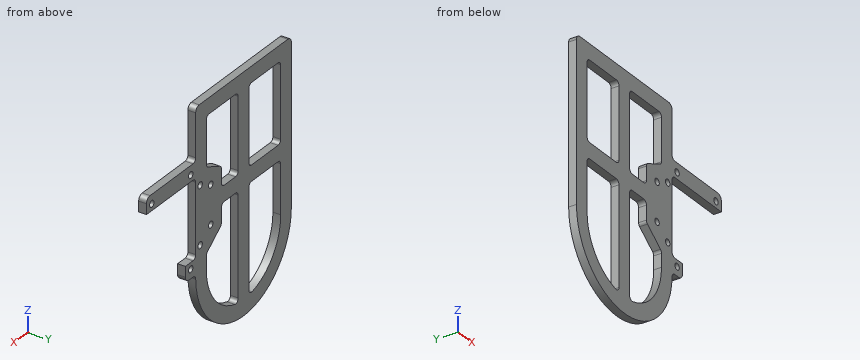
Autodesk Inventor part; units mm, degrees
ref_plane "YZ Plane" through (0, 0, 0) normal (1, 0, 0) x (0, 1, 0)
ref_plane "XZ Plane" through (0, 0, 0) normal (0, 1, 0) x (-1, 0, 0)
ref_plane "XY Plane" through (0, 0, 0) normal (0, 0, 1) x (1, 0, 0)
sketch "Sketch1" plane through (0, 0, 0) normal (0, 1, 0) x (-1, 0, 0)
  line L0 (0, 0) -> (0, -14.8)
  line L1 (0, -14.8) -> (-5.8, -14.8)
  line L2 (-5.8, -14.8) -> (-5.8, -20.8)
  line L3 (-5.8, -20.8) -> (0, -20.8)
  line L4 (0, 0) -> (0, 14.8)
  line L5 (0, 14.8) -> (-27.8, 14.8)
  line L6 (-27.8, 14.8) -> (-27.8, 20.8)
  line L7 (-27.8, 20.8) -> (0, 20.8)
  line L8 (0, 20.8) -> (0, 40.8)
  line L9 (0, 40.8) -> (54, 40.8)
  line L10 (0, -20.8) -> (0, -21.8)
  line L11 (54, 40.8) -> (54, -21.8)
  arc A0 (0, -21.8) -> (54, -21.8) centre (27, -21.8) ccw
  line L12 (-27.8, 17.3) -> (2.5, 17.3) construction
  line L13 (2.5, 17.3) -> (2.5, -17.3) construction
  line L14 (2.5, -17.3) -> (-5.8, -17.3) construction
  line L15 (0, 0) -> (2.5, 0) construction
  line L16 (2.5, 0) -> (8.5, 0) construction
  line L17 (8.5, -6.35) -> (8.5, 8.35) construction
  line L18 (-27.8, 14.8) -> (-5.8, -14.8) construction
  line L19 (-16.8, 0) -> (-21.8, 0) construction
  point P0 (-2.8, -17.3)
  point P1 (-2.8, 17.3)
  point P2 (-24.8, 17.3)
  point P3 (2.5, 11)
  point P4 (2.5, -11)
  dimension "d0" = 20
  dimension "d1" = 6
  dimension "d2" = 6
  dimension "d4" = 54
  dimension "d5" = 1
  dimension "d7" = 2.5
  dimension "d8" = 2.5
  dimension "d9" = 5.3
  dimension "d10" = 3
  dimension "d11" = 34.6
  dimension "d12" = 11
  dimension "d13" = 11
  dimension "d14" = 5.3
  dimension "d15" = 22
  dimension "d16" = 3
  dimension "d19" = 6
  dimension "d20" = 14.7
  dimension "d21" = 6.35
  dimension "d53" = 5
extrude "Extrusion1" add sketch "Sketch1" along normal blind 3
hole "Hole1" at (2.8, 0, -17.3) at (2.8, 0, 17.3) at (24.8, 0, 17.3) at (-2.5, 0, 11) at (-2.5, 0, -11) at (-8.5, 0, 8.35) at (-8.5, 0, -6.35) direction (0, 1, 0) diameter 2.5 end through all
fillet "ManufacturingFillet" radius 1.5 4 edges at (0, 1.5, -20.8) (0, 1.5, -14.8) (0, 1.5, 14.8) (0, 1.5, 20.8)
fillet "Fillet2" radius 2 4 edges at (5.8, 1.5, -20.8) (27.8, 1.5, 20.8) (0, 1.5, 40.8) (-54, 1.5, 40.8)
sketch "InteriorSketch" plane through (0, 3, 0) normal (0, 1, 0) x (1, 0, 0)
  arc A0 (-54, -38.8) -> (-52, -40.8) centre (-52, -38.8) ccw
  line L0 (-52, -40.8) -> (-2, -40.8)
  arc A1 (-2, -40.8) -> (0, -38.8) centre (-2, -38.8) ccw
  line L1 (0, -38.8) -> (0, -22.3)
  arc A2 (1.5, -20.8) -> (0, -22.3) centre (1.5, -22.3) ccw
  line L2 (1.5, -20.8) -> (25.8, -20.8)
  arc A3 (25.8, -20.8) -> (27.8, -18.8) centre (25.8, -18.8) ccw
  line L3 (27.8, -18.8) -> (27.8, -14.8)
  line L4 (27.8, -14.8) -> (1.5, -14.8)
  arc A4 (0, -13.3) -> (1.5, -14.8) centre (1.5, -13.3) ccw
  line L5 (0, -13.3) -> (0, 13.3)
  arc A5 (1.5, 14.8) -> (0, 13.3) centre (1.5, 13.3) ccw
  line L6 (1.5, 14.8) -> (5.8, 14.8)
  line L7 (5.8, 14.8) -> (5.8, 18.8)
  arc A6 (5.8, 18.8) -> (3.8, 20.8) centre (3.8, 18.8) ccw
  line L8 (3.8, 20.8) -> (1.4956, 20.8)
  arc A7 (-0.0042, 22.2737) -> (1.4956, 20.8) centre (1.4956, 22.3) ccw
  arc A8 (-0.0042, 22.2737) -> (-54, 21.8) centre (-27, 21.8) ccw
  line L9 (-54, 21.8) -> (-54, -38.8)
  circle A9 centre (-8.5, -8.35) radius 1.25
  circle A10 centre (-2.5, -11) radius 1.25
  circle A11 centre (2.8, -17.3) radius 1.25
  circle A12 centre (2.8, 17.3) radius 1.25
  circle A13 centre (24.8, -17.3) radius 1.25
  circle A14 centre (-2.5, 11) radius 1.25
  circle A15 centre (-8.5, 6.35) radius 1.25
  line L10 (-14.5, 9.2909) -> (-14.5, -12.2592)
  line L11 (-14.5, -12.2592) -> (-6, -16.0133)
  line L12 (-6, -16.0133) -> (-6, -34.8)
  line L13 (-6, -34.8) -> (-48, -34.8)
  circle A16 centre (-2.5, 11) radius 1.25 construction
  line L14 (-8.5, 6.35) -> (-2.5, 11) construction
  line L15 (-8.5, -8.35) -> (-2.5, -11) construction
  line L16 (-14.5, 9.2909) -> (-6, 15.8784)
  line L17 (-6, 15.8784) -> (-6, 21.8)
  line L18 (-6, 15.8784) -> (-6, 21.8)
  arc A17 (-6, 21.8) -> (-48, 21.8) centre (-27, 21.8) ccw
  line L19 (-48, 21.8) -> (-48, -34.8)
  line L20 (-6, 21.8) -> (-48, 21.8) construction
  line L21 (-27, -34.8) -> (-27, 42.8) construction
  line L22 (-14.5, -1.4841) -> (-48, -1.4841) construction
  line L23 (-14.5, 1.5159) -> (-24, 1.5159)
  line L24 (-24, 1.5159) -> (-24, 42.5846)
  line L25 (-30, 42.5846) -> (-30, 1.5159)
  line L26 (-30, 1.5159) -> (-48, 1.5159)
  line L27 (-48, -4.4841) -> (-30, -4.4841)
  line L28 (-30, -4.4841) -> (-30, -34.8)
  line L29 (-14.5, -4.4841) -> (-24, -4.4841)
  line L30 (-24, -4.4841) -> (-24, -34.8)
  line L31 (-30, 1.5159) -> (-24, 1.5159) construction
  line L32 (-30, 1.5159) -> (-30, -4.4841) construction
  point P0 (0, 0)
  point P1 (-14.5, -1.4841)
  point P2 (-27, -1.4841)
  point P3 (-30, -1.4841)
  point P4 (-27, 1.5159)
  dimension "d31" = 6
  dimension "d32" = 6
  dimension "d34" = 6
  dimension "d38" = 6
  dimension "d39" = 6
  dimension "d44" = 6
  dimension "d48" = 6
  dimension "d49" = 6
extrude "Extrusion3" cut sketch "InteriorSketch" against normal through all contours L10 L23 L24 A17 L17 L16 | L10 L11 L12 L13 L30 L29 | L25 L26 L19 A17 | L13 L19 L27 L28
fillet "Fillet3" radius 1.5 18 edges at (-24, 1.5, 34.8) (-6, 1.5, 34.8) (-24, 1.5, 4.4841) (-14.5, 1.5, 4.4841) (-6, 1.5, 16.0133) (-14.5, 1.5, 12.2592) (-14.5, 1.5, -9.2909) (-6, 1.5, -15.8784) (-24, 1.5, -42.5846) (-14.5, 1.5, -1.5159) (-24, 1.5, -1.5159) (-30, 1.5, -1.5159) (-30, 1.5, 4.4841) (-30, 1.5, 34.8) (-48, 1.5, 34.8) (-48, 1.5, 4.4841) (-48, 1.5, -1.5159) (-30, 1.5, -42.5846)
ref_plane "Work Plane3" through (19, 0, 13.3) normal (1, 0, 0) x (0, 0, -1)
ref_plane "Work Plane4" through (27.8, 0, -5.2) normal (0, 0, -1) x (-1, 0, 0)
equation "\"d0\" = head_back_length"
equation "\"d1\" = fix_width"
equation "\"d2\" = fix_width"
equation "\"d4\" = head_height"
equation "\"d5\" = head_forward - 0.5 * head_height"
equation "\"d7\" = hole_2_intern"
equation "\"d8\" = hole_2_intern"
equation "\"d11\" = side_2_side_hole"
equation "\"d19\" = camera_holes_offset_z"
equation "\"d20\" = camera_holes_dist"
equation "\"d21\" = 0.5 * camera_holes_dist - camera_holes_offset_x"
equation "\"d17\" = plate_thickness"
equation "\"d31\" = structure_width"
equation "\"d32\" = structure_width"
equation "\"d34\" = structure_width"
equation "\"d38\" = structure_width"
equation "\"d39\" = structure_width"
equation "\"d44\" = structure_width"
equation "\"d48\" = structure_width"
equation "\"d49\" = structure_width"
equation "\"head_back_length\" = 20"
equation "\"head_height\" = 54"
equation "\"head_forward\" = 28"
equation "\"fix_width\" = 6"
equation "\"fix_2_fix\" = 29.1"
equation "\"hole_2_intern\" = hole_2_servo - fix_2_servo_margin"
equation "\"fix_2_servo_margin\" = 0.3"
equation "\"hole_2_servo\" = 2.8"
equation "\"side_2_side_hole\" = 34.6"
equation "\"hole_side_2_hole_top\" = 5.3"
equation "\"hole_2_extern\" = 3"
equation "\"hole_2_hole\" = 22"
equation "\"plate_thickness\" = 3"
equation "\"camera_holes_offset_z\" = 6"
equation "\"camera_holes_dist\" = 14.7"
equation "\"camera_holes_offset_x\" = 1"
equation "\"structure_width\" = 6"
properties part number "base_head" material "Aluminum 6061"
Input: part model. Units: mm. Frame: model coordinates. Round coordinates to 2 decimals unless told otherwise and drop trailing zeros. Write each loop counter-clockwise with the first axis right and the second up, starting at its lowest first coordinate (ties: lowest second). Pieces come first, ordered by that corner, then holes. Notation, with made-up numbers: (-40, -15.75) -> (6, -15.75) arc R13 cw to (6, 2.25) -> close; hole circle Ø10 at (88, 43.25). An arc over 180 degrees is marked (long way). Answer as CSV lines item,"result".
1. Section C-C (y = 0.55). Give the number of separate pieces and of enclosed holes in the cut face, plus the area to 3 significant figures.
Geometry says:
separate pieces,"1"
enclosed holes,"11"
area,"2,490 mm^2"
2. Contact query for flat-ended pins moving along their axis: P1, Ø0.9, axis at y = 1.5, z = -23, coming from the -X side; P2, Ø1, axis at x = -34.5, y = 1, coming from the -Z side; P3, Ø1.5, axis at x = 4, y = 2, coming from the +Z side. Output: stop coordinate, or through.
Geometry says:
P1,"stops at x = -53.99"
P2,"stops at z = -47.88"
P3,"stops at z = 20.8"
3. Ray query, L1, parallel to Z at x = 2.8, y = 2.2; L2, parallel to X at y = 2.3, z = 8.35; L3, parallel to X at y = 1.2, z = 17.3. Return the intervals inside material, ascending. Write a range as [from, to].
Geometry says:
L1,"z = [-20.8, -18.55], [-16.05, -14.8], [14.8, 16.05], [18.55, 20.8]"
L2,"x = [-54, -48], [-30, -24], [-14.5, -9.75], [-7.25, 0]"
L3,"x = [-54, -48], [-30, -24], [-6, 1.55], [4.05, 23.55], [26.05, 27.8]"
4. Section A-A (z = -6.35). Return the cut outline in (x, y).
Geometry says:
outline,"(-54, 0) -> (-48, 0) -> (-48, 3) -> (-54, 3) -> close; (-30, 0) -> (-24, 0) -> (-24, 3) -> (-30, 3) -> close; (-14.5, 0) -> (-9.75, 0) -> (-9.75, 3) -> (-14.5, 3) -> close; (-7.25, 0) -> (0, 0) -> (0, 3) -> (-7.25, 3) -> close"
5. Section D-D (x = 19). Return the cut outline in (y, z).
Geometry says:
outline,"(0, 14.8) -> (3, 14.8) -> (3, 20.8) -> (0, 20.8) -> close"
6. Section B-B (x = -11). Return the cut outline in (y, z) (3 decimals).
Geometry says:
outline,"(0, -43.549) -> (3, -43.549) -> (3, -35.401) -> (0, -35.401) -> close; (0, -12.003) -> (3, -12.003) -> (3, 13.805) -> (0, 13.805) -> close; (0, 34.8) -> (3, 34.8) -> (3, 40.8) -> (0, 40.8) -> close"
